The drawing under review shows one solid part. Ordinate dimensions are in mm from its lowest x, y, z. Round coordinates to 2 decimals unless told otherwise and drop trailing zeros. Order: outer loops, then holes, each group sorted by start corner. A loop starts at its lowest first (then second) coordinate and runs counter-clockwise, first axis right, second up. Notation, with made-up numbers: M -29.75,-0.5 L 17.25,-0.5 A22 cw 17.25,30.5 Z; hole C -16.75,69 d10. An arc over 180 degrees is marked long. Use a Markdown table: item, result.
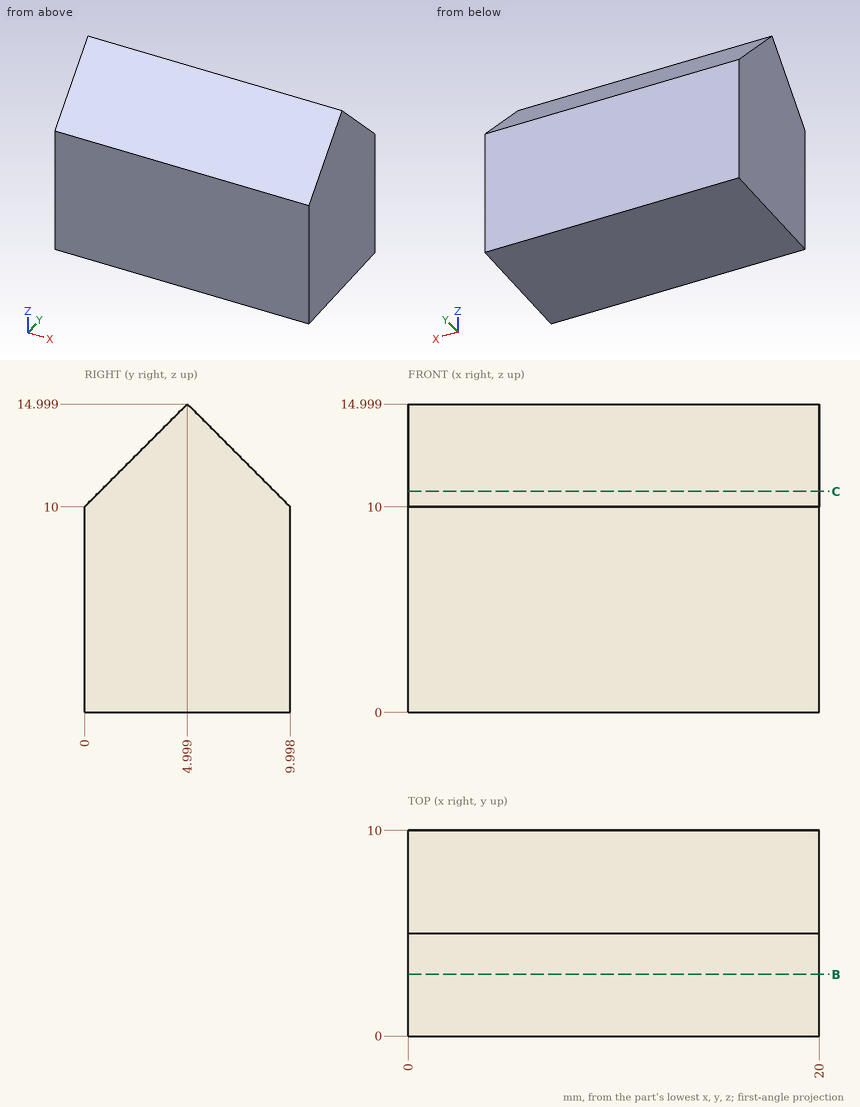
Q1. Clearance check with a flat-ended pin moving along its axis: pin 1 (1 mm diameter, centred on x = 4, y = 4, fed in from +Z). State where the tip first meets the part, or that it passes through.
Determined:
| item | result |
|---|---|
| pin 1 | stops at z = 14.5 |
Q2. Add section B-B (y = 3). Write out the cut boundary in (x, z), then the cut area to 3 significant figures.
Determined:
| item | result |
|---|---|
| outline | M 0,0 L 20,0 L 20,13 L 0,13 Z |
| area | 260 mm^2 |
Q3. Wall thickness on line 1 along Z through (x, y) = (3, 4.75); line 2 along Z through (x, y) = (6, 7.5); line 3 along Y through (x, z) = (5, 10.5): over which ranges is each line inside the solid? List them lowest first. Write a range as [from, to].
Determined:
| item | result |
|---|---|
| line 1 | z = [0, 14.75] |
| line 2 | z = [0, 12.5] |
| line 3 | y = [0.5, 9.5] |
Q4. Add section C-C (z = 10.75). Write out the cut boundary in (x, y), then the cut area to 3 significant figures.
Determined:
| item | result |
|---|---|
| outline | M 0,0.75 L 20,0.75 L 20,9.25 L 0,9.25 Z |
| area | 170 mm^2 |
